Design review of the part built by this model. Coordinates are the model's own, in mm. Face numbers are marked on the shaded views. Round coordinates to 2 decimals unless told otherwise and drop trailing zeros. Order: outer loops, then holes, each group sorted by start corner. A loop starts at its lowest first (then second) coordinate and runs counter-clockwise, first axis right, second up. Notation, with made-up numbers: (86.25, 63) - (95.25, 63) arc R24 ccw to (95.25, 84) - close; hole circle Ø4 at (46.25, 71). An arc over 180 degrees is marked (long way). Answer as a JSON object with one key per item and string values. Group by question number.
from build123d import *

# Parameters (mm, degrees)
F0_W        = 175
F0_H        = 143
F1_DEPTH    = 2.5
F2_W        = 170
F2_H        = 138.5
F3_DEPTH    = 6
F4_T        = 2.5
F4_T3_DEPTH = 175
F4_T5_DEPTH = 143.5


# Not quite as in the source:
# - a shell that OpenCascade refuses in one call is made with other operations: the cavity is built on its own and cut out


with BuildPart() as f1:
    # F0 (on Front) → F1 (new body)
    with BuildSketch(Plane.XZ):
        Rectangle(F0_W, F0_H)
    extrude(amount=F1_DEPTH)

    # F2 (on face) → F3 (join)
    with BuildSketch(Plane.XZ.offset(2.5)):
        Rectangle(F2_W, F2_H)
    extrude(amount=F3_DEPTH)

    # F4: shell of thickness 2.5, made by hand


with BuildPart() as f4_core1:
    # F4_t2: copy of F1
    add(f1.part)

    # the walls: a layer under each face that stays
    f4_faces = [f4_core1.faces().sort_by_distance(p)[0] for p in [
        (0, -1.25, -71.5),
        (-87.5, -1.25, 0),
        (87.5, -1.25, 0),
        (0, 0, 0),
        (60.15625, -2.5, -69.7345679012),
        (0, -1.25, 71.5),
        (0, -5.5, -69.25),
        (85, -5.5, 0),
        (0, -5.5, 69.25),
        (-85, -5.5, 0),
    ]]
    thicken(f4_faces, amount=-F4_T, mode=Mode.SUBTRACT)

    # F4_s4 → F4_t3 (cut)
    with BuildSketch(Plane.YZ.offset(-87.5)):
        Polygon((-2.525, -69.275), (0, -69.25), (0, -66.75), (-2.5, -66.75), align=None)
        Polygon((-2.525, 69.275), (0, 69.25), (0, 66.75), (-2.5, 66.75), align=None)
    extrude(amount=F4_T3_DEPTH, mode=Mode.SUBTRACT)

    # F4_s6 → F4_t5 (cut)
    with BuildSketch(Plane.XY.offset(-71.75)):
        Polygon((85.025, -2.525), (85, 0), (82.5, 0), (82.5, -2.5), align=None)
        Polygon((-85.025, -2.525), (-85, 0), (-82.5, 0), (-82.5, -2.5), align=None)
    extrude(amount=F4_T5_DEPTH, mode=Mode.SUBTRACT)


with BuildPart() as f1_1:
    add(f1.part)

    # what is left inside the walls is the cavity
    f4_cavity = [f4_core1.part.solids().sort_by_distance(p)[0] for p in [
        (0, -2.525, -22.25),
    ]]
    add(f4_cavity, mode=Mode.SUBTRACT)


solid = f1_1.part
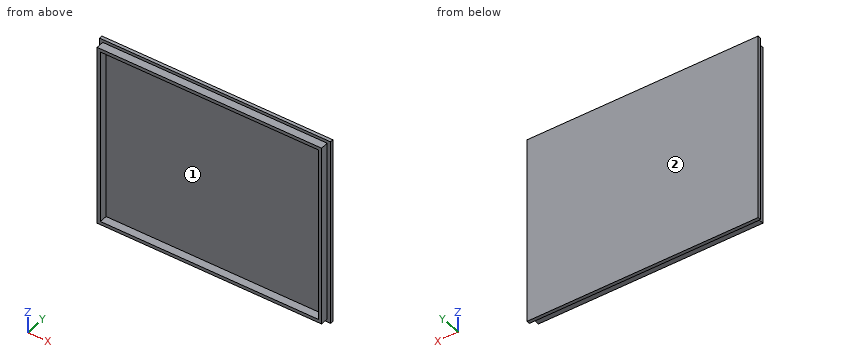
1. Take a section at B-B, the plane x = 27. Give the boundary of the cut face in (y, z), then the cut area to 4 significant figures.
2. Clearance check with flat-ended pins moving along their axes: P1, Ø1.8, axis at x = -41, y = -5, coming from the +Z side; P2, Ø2, axis at y = -7, z = -37.5, coming from the -X side; P3, Ø1.8, axis at x = 7.5, y = -5, coming from the -Z side; P4, Ø5, axis at y = -4, z = -27.5, coming from the -X side. State where each tip first meets the part, or that it passes through.
3. Mouldability with a two-part tool opening along Z and no side actions: class the marked faces 1 and 2 as pulls with the +Z half, pulls with the -Z half, needs draft (parallel to the pull), parting line crosses it, or undercut.
4. Take a section at A-A, the plane y = -4.25. Give the boundary of the cut face in (x, z), then the cut area to 3 significant figures.
5. To check wall thickness, follow line 1 (Z direction, x = 33, y = -4.5); line 2 (X direction, y = -4, z = -13); line 3 (Y direction, x = 59, z = -60). State the ranges of each line that lie inside material, in increasing order. Write a range as from..to.
6. Take a section at C-C, the plane z = 33. Give the boundary of the cut face in (x, y).
Response values:
{
 "1": {"outline": "(-8.5, -69.25) - (-2.5, -69.25) - (-2.5, -71.5) - (0, -71.5) - (0, 71.5) - (-2.5, 71.5) - (-2.5, 69.25) - (-8.5, 69.25) - (-8.5, 66.75) - (-2.5, 66.75) - (-2.5, -66.75) - (-8.5, -66.75) - close", "area": "387.5 mm2"},
 "2": {"P1": "z = 69.25", "P2": "x = -85", "P3": "z = -69.25", "P4": "x = -87.5"},
 "3": {"face 1": "undercut", "face 2": "needs draft"},
 "4": {"outline": "(-85, -69.25) - (85, -69.25) - (85, 69.25) - (-85, 69.25) - close; hole (-82.5, -66.75) - (82.5, -66.75) - (82.5, 66.75) - (-82.5, 66.75) - close", "area": "1,520 mm2"},
 "5": {"line 1": "-69.25..-66.75, 66.75..69.25", "line 2": "-85..-82.5, 82.5..85", "line 3": "-2.5..0"},
 "6": {"outline": "(-87.5, -2.5) - (-85, -2.5) - (-85, -8.5) - (-82.5, -8.5) - (-82.5, -2.5) - (82.5, -2.5) - (82.5, -8.5) - (85, -8.5) - (85, -2.5) - (87.5, -2.5) - (87.5, 0) - (-87.5, 0) - close"}
}
